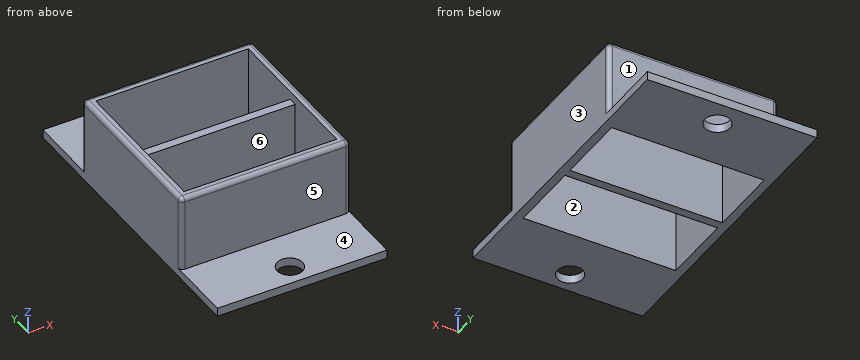
from build123d import *

# Parameters (mm, degrees)
F0_W     = 20
F0_H     = 20
F1_DEPTH = 10
F2_T     = -1
F4_DEPTH = 9
F5_W     = 20
F5_H     = 8
F5_R     = 1.5
F6_DEPTH = 1
F7_W     = 18
F7_H     = 18
F8_DEPTH = 1
F9_R     = 0.5


with BuildPart() as f1:
    # F0 (on Top) → F1 (new body)
    with BuildSketch(Plane.XY):
        Rectangle(F0_W, F0_H)
    extrude(amount=F1_DEPTH)

    # F2
    f2_openings = [f1.faces().sort_by_distance(p)[0] for p in [
        (0, 0, 0),
    ]]
    offset(amount=F2_T, openings=f2_openings)

    # F3 (on Top) → F4 (join)
    with BuildSketch(Plane.XY):
        Polygon((9, -0.5), (9, 0.5), (0.5, 0.5), (-0.5, 0.5), (-9, 0.5), (-9, -0.5), (-0.5, -0.5), (0.5, -0.5), align=None)
    extrude(amount=F4_DEPTH)

    # F5 (on Top) → F6 (join)
    with BuildSketch(Plane.XY):
        with Locations((0, -13.5)):
            Rectangle(F5_W, F5_H)
        with Locations((0, -15)):
            Circle(F5_R, mode=Mode.SUBTRACT)
        with Locations((0, 14)):
            Rectangle(F5_W, F5_H)
        with Locations((0, 15)):
            Circle(F5_R, mode=Mode.SUBTRACT)
    extrude(amount=F6_DEPTH)

    # F7 (on face) → F8 (cut)
    with BuildSketch(Plane.XY.offset(10)):
        Rectangle(F7_W, F7_H)
    extrude(amount=-F8_DEPTH, mode=Mode.SUBTRACT)

    # F9
    f9_edges = [f1.edges().sort_by_distance(p)[0] for p in [
        (-10, -10, 5.5),
        (10, -10, 5.5),
        (0, -10, 10),
        (10, 0, 10),
        (-10, 0, 10),
        (10, 10, 5.5),
        (-10, 10, 5.5),
        (0, 10, 10),
    ]]
    fillet(f9_edges, radius=F9_R)


solid = f1.part
Read the model definition and answer for the solid it produces. Units are mm, in the model's axes. Face numbers are marked on the shaded views. A direction names the side the tool comes from. Round coordinates to 2 decimals unless told otherwise and drop trailing zeros. Write each loop counter-clockwise with the first axis right and the second up, starting at its lowest first coordinate (ties: lowest second). Pieces come first, ordered by that corner, then holes.
Q1. Find section D-D on z = 1.5. Determine the outline of the cut face in (x, y).
Values:
outline: (-10, -9.5) arc R0.5 ccw to (-9.5, -10) - (9.5, -10) arc R0.5 ccw to (10, -9.5) - (10, 9.5) arc R0.5 ccw to (9.5, 10) - (-9.5, 10) arc R0.5 ccw to (-10, 9.5) - close; hole (-9, -9) - (9, -9) - (9, -0.5) - (-9, -0.5) - close; hole (-9, 0.5) - (9, 0.5) - (9, 9) - (-9, 9) - close
Q2. Find section A-A on y = 15. Determine the outline of the cut face in (x, z).
Values:
outline: (-10, 0) - (-1.5, 0) - (-1.5, 1) - (-10, 1) - close; (1.5, 0) - (10, 0) - (10, 1) - (1.5, 1) - close
Q3. Find section C-C on x = 7.25. Determine the outline of the cut face in (y, z), and give its area (3 significant figures).
Values:
outline: (-17.5, 0) - (-9, 0) - (-9, 10) - (-9.5, 10) arc R0.5 ccw to (-10, 9.5) - (-10, 1) - (-17.5, 1) - close; (-0.5, 0) - (0.5, 0) - (0.5, 9) - (-0.5, 9) - close; (9, 0) - (18, 0) - (18, 1) - (10, 1) - (10, 9.5) arc R0.5 ccw to (9.5, 10) - (9, 10) - close
area: 44.4 mm2
Q4. A tool of negligible diameter and unlimited length cuts with its end or side. For the marked faces 1, 2 and 3, from which of +Z, -Z, +X, -X, +Y, -Y can it reach the whole face along a straight path? Write none if from no direction.
Values:
face 1: +Z, +X, -X, +Y
face 2: +Z, -Z
face 3: +Z, -Z, +X, +Y, -Y
Q5. The mould has two halves that part along Y. Classify the marked faces 4, 5 and 6: released by +Y, released by -Y, zero draft, split by the parting line, or undercut.
Values:
face 4: zero draft
face 5: released by -Y
face 6: undercut
Q6. Straight lines are drawn through the part: line 1 (Y direction, x = 0, z = 0.75); line 2 (Y direction, x = -4.5, z = 5.25); line 3 (Y direction, x = 5.25, z = 9.5). For each, find the intervals that lie inside material, in ascending order.
Values:
line 1: y = -17.5 to -16.5, -13.5 to -9, -0.5 to 0.5, 9 to 13.5, 16.5 to 18
line 2: y = -10 to -9, -0.5 to 0.5, 9 to 10
line 3: y = -10 to -9, 9 to 10
Q7. Find section B-B on x = 0. Determine the outline of the cut face in (y, z), and give its area (3 significant figures).
Values:
outline: (-17.5, 0) - (-16.5, 0) - (-16.5, 1) - (-17.5, 1) - close; (-13.5, 0) - (-9, 0) - (-9, 10) - (-9.5, 10) arc R0.5 ccw to (-10, 9.5) - (-10, 1) - (-13.5, 1) - close; (-0.5, 0) - (0.5, 0) - (0.5, 9) - (-0.5, 9) - close; (9, 0) - (13.5, 0) - (13.5, 1) - (10, 1) - (10, 9.5) arc R0.5 ccw to (9.5, 10) - (9, 10) - close; (16.5, 0) - (18, 0) - (18, 1) - (16.5, 1) - close
area: 38.4 mm2
Q8. Flat-ended cylindrical pins translate along their axes: P1, Ø6.5, axis at x = 3.5, y = -13.5, coming from the +Z side; P2, Ø3, axis at x = 5, z = 3.5, coming from the +Y side; P3, Ø2.5, axis at x = 4, z = 5.5, coming from the -Y side. Find the tip coordinate at first contact, or state that the pin passes through.
Values:
P1: stops at z = 1
P2: stops at y = 10
P3: stops at y = -10
